Design review of the part built by this model. Coordinates are the model's own, in mm. A direction names the side the tool comes from. Round coordinates to 2 decimals unless told otherwise and drop trailing zeros. Loops run counter-clockwise (first coordinate to the right, second up) from the corner with the lowest first, then second, coordinate; pieces in that order, holes last. Notation, with made-up numbers: M 12.5,65.25 L 56.5,65.25 A25 ccw 56.5,79.25 Z; hole C -24.5,-15.5 d5. An arc over 180 degrees is marked long. Use a Markdown table: item, result.
from build123d import *

# Parameters (mm, degrees)
SKETCH1_R           = 38.1
SKETCH1_W           = 38.0365
SKETCH1_H           = 12.7508
BOSS_EXTRUDE1_DEPTH = 5.6642
SKETCH1_3_R         = 38.1
SKETCH1_3_W         = 38.0365
SKETCH1_3_H         = 12.7508
SKETCH1_3_R_2       = 3.71475
BOSS_EXTRUDE2_DEPTH = 5.715
BOSS_EXTRUDE3_DEPTH = 15.875
CUT_EXTRUDE2_DEPTH  = 59.02721


with BuildPart() as part:
    # Sketch1 → Boss-Extrude1 (new body)
    with BuildSketch(Plane(origin=(0, 0, 0), x_dir=(1, 0, 0), z_dir=(0, 1, 0))):
        with Locations(Location((0, 0, 0), (0, 0, 90))):
            Circle(SKETCH1_R)
        Rectangle(SKETCH1_W, SKETCH1_H, mode=Mode.SUBTRACT)
    extrude(amount=BOSS_EXTRUDE1_DEPTH)

    # Sketch1_3 → Boss-Extrude2 (add)
    with BuildSketch(Plane(origin=(0, 0, 0), x_dir=(1, 0, 0), z_dir=(0, 1, 0))):
        with Locations(Location((0, 0, 0), (0, 0, 90))):
            Circle(SKETCH1_3_R)
        Rectangle(SKETCH1_3_W, SKETCH1_3_H, mode=Mode.SUBTRACT)
        Rectangle(SKETCH1_3_W, SKETCH1_3_H)
        with Locations(Location((0, 0, 0), (0, 0, 270))):
            Circle(SKETCH1_3_R_2, mode=Mode.SUBTRACT)
    extrude(amount=-BOSS_EXTRUDE2_DEPTH)

    # Sketch2 → Boss-Extrude3 (add, symmetric)
    with BuildSketch(Plane(origin=(0, 0, 0), x_dir=(1, 0, 0), z_dir=(0, 1, 0))):
        with BuildLine():
            ThreePointArc((28.608885, -20.032157), (16.12657, -30.978853), (0, -34.925))
            Line((0, -34.925), (0, -38.1))
            ThreePointArc((0, -38.1), (17.592622, -33.795113), (31.209693, -21.853262))
            Line((31.209693, -21.853262), (28.608885, -20.032157))
        make_face()
        with BuildLine():
            Line((0, -38.1), (0, -34.925))
            ThreePointArc((0, -34.925), (-16.12657, -30.978853), (-28.608885, -20.032157))
            Line((-28.608885, -20.032157), (-31.209693, -21.853262))
            ThreePointArc((-31.209693, -21.853262), (-17.592622, -33.795113), (0, -38.1))
        make_face()
        with BuildLine():
            Line((0, 34.925), (0, 38.1))
            ThreePointArc((0, 38.1), (-13.030967, 35.802289), (-24.490208, 29.186293))
            Line((-24.490208, 29.186293), (-22.449357, 26.754102))
            ThreePointArc((-22.449357, 26.754102), (-11.945054, 32.818765), (0, 34.925))
        make_face()
        with BuildLine():
            ThreePointArc((24.490208, 29.186293), (13.030967, 35.802289), (0, 38.1))
            Line((0, 38.1), (0, 34.925))
            ThreePointArc((0, 34.925), (11.945054, 32.818765), (22.449357, 26.754102))
            Line((22.449357, 26.754102), (24.490208, 29.186293))
        make_face()
    extrude(amount=BOSS_EXTRUDE3_DEPTH, both=True)

    # Sketch3 → Cut-Extrude2 (cut, through all)
    with BuildSketch(Plane(origin=(0, 5.6642, 0), x_dir=(1, 0, 0), z_dir=(0, 1, 0))):
        with BuildLine():
            Line((-19.0754, 16.5354), (19.0754, 16.5354))
            ThreePointArc((19.0754, 16.5354), (0, 25.163724), (-19.0754, 16.5354))
        make_face()
        with BuildLine():
            Line((-19.0754, -16.5354), (19.0754, -16.5354))
            ThreePointArc((19.0754, -16.5354), (0, -25.163724), (-19.0754, -16.5354))
        make_face()
    extrude(amount=-CUT_EXTRUDE2_DEPTH, mode=Mode.SUBTRACT)


solid = part.part
1. The part is to be moulded in two halves that separate along X. For faces 1 (the face through (-29.89, -10.87, 20.93)), 2 (the face through (-1, 5.664, -7)), 3 (the face through (-1.9, 15.875, -35.4)), say which applies: pulls with the +X half, pulls with the -X half, needs draft (parallel to the pull), parting line crosses it, or undercut.
Check values:
| item | result |
|---|---|
| face 1 | pulls with the -X half |
| face 2 | undercut |
| face 3 | needs draft |
2. Machinability: for faces 4 (the face through (-1, -5.715, -7)), 5 (the face through (-23.484, -10.724, -27.987)), 6 (the face through (29.927, -10.866, 20.955)), 7 (the face through (-23.484, 10.841, -27.987)), which of the approach directions +Z, -Z, +X, -X, +Y, -Y give a long, thin tool a straight path to every point of the face, cutting with its end or side? Answer none if there is none.
Check values:
| item | result |
|---|---|
| face 4 | -Y |
| face 5 | -X, -Y |
| face 6 | -Z, +X, -Y |
| face 7 | -X, +Y |
3. Take a section at A-A on y = 8. Give the boundary of the cut face in (x, z) (3 decimals), and give its area (3 significant figures).
Check values:
| item | result |
|---|---|
| outline | M -31.21,21.853 L -28.609,20.032 A34.925 cw 0,34.925 A34.925 cw 28.609,20.032 L 31.21,21.853 A38.1 ccw 0,38.1 A38.1 ccw Z; M -24.49,-29.186 A38.1 ccw 24.49,-29.186 L 22.449,-26.754 A34.925 cw 0,-34.925 A34.925 cw -22.449,-26.754 Z |
| area | 384 mm² |
4. Insertion check: pin 1 (8 mm diameter, centred on y = -7, z = -18.5, fed in from +X); pin 2 (3 mm diameter, centred on y = 2.5, z = 0.5, fed in from -X); pin 3 (3 mm diameter, centred on x = -9, y = 3, fed in from +Z). Each pin has a flat end and moves straight along its axis. Give the tip position at first contact, or say it passes through.
Check values:
| item | result |
|---|---|
| pin 1 | stops at x = 35.14 |
| pin 2 | stops at x = -38.1 |
| pin 3 | stops at z = 37.35 |
5. Wall thickness on line 1 along X through (y, z) = (-2.45, 0); line 2 along Z through (x, y) = (17.5, -2.5); line 3 along Z through (x, y) = (8, -3): over which ranges is each line inside the solid? List them lowest first. Write a range as from..to.
Check values:
| item | result |
|---|---|
| line 1 | x = -38.1..-3.71, 3.71..38.1 |
| line 2 | z = -33.84..-18.17, -16.54..16.54, 18.17..33.84 |
| line 3 | z = -37.25..-23.87, -16.54..16.54, 23.87..37.25 |
6. Take a section at D-D on x = -10.5. Give the boundary of the cut face in (y, z) (3 decimals).
Check values:
| item | result |
|---|---|
| outline | M -15.875,-36.625 L 15.875,-36.625 L 15.875,-33.309 L 5.664,-33.309 L 5.664,-22.892 L -5.715,-22.892 L -5.715,-33.309 L -15.875,-33.309 Z; M -15.875,33.309 L -5.715,33.309 L -5.715,22.892 L 5.664,22.892 L 5.664,33.309 L 15.875,33.309 L 15.875,36.625 L -15.875,36.625 Z; M -5.715,-16.535 L 5.664,-16.535 L 5.664,-6.375 L 0,-6.375 L 0,6.375 L 5.664,6.375 L 5.664,16.535 L -5.715,16.535 Z |
7. Take a section at C-C on y = 2. Give the boundary of the cut face in (x, z).
Check values:
| item | result |
|---|---|
| outline | C 0,0 d76.2; hole M -19.08,-16.54 A25.4 ccw 19.08,-16.54 Z; hole M -19.08,16.54 L 19.08,16.54 A25.4 ccw Z; hole M -19.02,-6.38 L 19.02,-6.38 L 19.02,6.38 L -19.02,6.38 Z |
8. Take a section at B-B on z = 0. Give the boundary of the cut face in (x, y) (3 decimals), and give its area (3 significant figures).
Check values:
| item | result |
|---|---|
| outline | M -38.1,-5.715 L -3.715,-5.715 L -3.715,0 L -19.018,0 L -19.018,5.664 L -38.1,5.664 Z; M 3.715,-5.715 L 38.1,-5.715 L 38.1,5.664 L 19.018,5.664 L 19.018,0 L 3.715,0 Z |
| area | 609 mm² |
